Could you check a few things on this model? Use its own coordinates, in mm. A direction names the side the tool comes from. Give positions to 0.01 mm unless a question says otherwise; leave off trailing zeros. Loops run counter-clockwise (first coordinate to the right, second up) from the corner with the lowest first, then second, coordinate; pieces in that order, holes last.
1. I need wall thicknesses on line 1 along Y through (x, z) = (119.5, 2.95); line 2 along Y through (x, z) = (17, 3.8); line 3 along X through (y, z) = (14.75, 4.1). Which ranges of each line are inside material? Lowest first, please.
2. Thinking about a two-plate mould opening in Y: for faces 4 (the flat face through (63, 30, 2)), 5 (the flat face through (125, 2, 2)), 6 (the flat face through (5, 5, 2)), which applies, +Y half, -Y half, draft (parallel to the pull), parting line (faces both ways), or undercut?
3. Imagine slicing it at C-C (y = 15). List the corners of the cut face in (x, z) for me.
4. Imagine slicing it at D-D (x = 11.5). List the corners of the cut face in (y, z) for me.
5. Imagine slicing it at A-A (x = 117). List the corners of the cut face in (y, z) for me.
6. Imagine slicing it at B-B (z = 3.2). List the corners of the cut face in (x, y) for me, plus the area to 3 significant figures.
7. For P1, Ø8, axis at x = 59.5, y = 4.5, coming from the -Z side; P2, Ø1.5, axis at y = 12.5, z = 2.5, coming from the -X side, each with a flat end and sliding along its axis, tell me the tip position at first contact or that it passes through.
8. For faces 1 (the flat face through (62, 15, 5)), 2 (the flat face through (120, 5, 2)), 3 (the flat face through (5, 25, 2)), which set-ups out of +Z, -Z, +X, -X, +Y, -Y let a thin tool reach every point of the face, with its end or its side?
Autodesk Inventor part; units mm, degrees
ref_plane "YZ Plane" through (0, 0, 0) normal (1, 0, 0) x (0, 1, 0)
ref_plane "XZ Plane" through (0, 0, 0) normal (0, 1, 0) x (-1, 0, 0)
ref_plane "XY Plane" through (0, 0, 0) normal (0, 0, 1) x (1, 0, 0)
sketch "スケッチ1" plane through (0, 0, 0) normal (0, 0, 1) x (1, 0, 0)
  line L0 (0, 0) -> (125, 0)
  line L1 (125, 30) -> (0, 30)
  arc A0 (10, 5) -> (10, 25) centre (10, 15) ccw
  arc A1 (115, 25) -> (115, 5) centre (115, 15) ccw
  line L2 (10, 25) -> (0, 25)
  line L3 (10, 5) -> (0, 5)
  line L4 (115, 25) -> (125, 25)
  line L5 (115, 5) -> (125, 5)
  line L6 (0, 30) -> (0, 25)
  line L7 (0, 5) -> (0, 0)
  line L8 (125, 0) -> (125, 5)
  line L9 (125, 25) -> (125, 30)
  dimension "d0" = 125
  dimension "d1" = 30
  dimension "d2" = 20
  dimension "d3" = 20
  dimension "d7" = 125
  dimension "d9" = 5
  dimension "d12" = 10
  dimension "d15" = 115
extrude "押し出し1" add sketch "スケッチ1" along normal blind 5
properties part number "RescueKit-Slide"
Derived:
1. line 1: y = 0 to 5, 25 to 30
1. line 2: y = 0 to 7.86, 22.14 to 30
1. line 3: x = 20 to 105
2. face 4: +Y half
2. face 5: draft
2. face 6: undercut
3. outline: (20, 0) - (105, 0) - (105, 5) - (20, 5) - close
4. outline: (0, 0) - (5.11, 0) - (5.11, 5) - (0, 5) - close; (24.89, 0) - (30, 0) - (30, 5) - (24.89, 5) - close
5. outline: (0, 0) - (5, 0) - (5, 5) - (0, 5) - close; (25, 0) - (30, 0) - (30, 5) - (25, 5) - close
6. outline: (0, 0) - (125, 0) - (125, 5) - (115, 5) arc R10 cw to (115, 25) - (125, 25) - (125, 30) - (0, 30) - (0, 25) - (10, 25) arc R10 cw to (10, 5) - (0, 5) - close
6. area: 3,040 mm2
7. P1: stops at z = 0
7. P2: stops at x = 19.46
8. face 1: +Z, +X, -X, +Y, -Y
8. face 2: +Z, -Z, +X
8. face 3: +Z, -Z, -X
